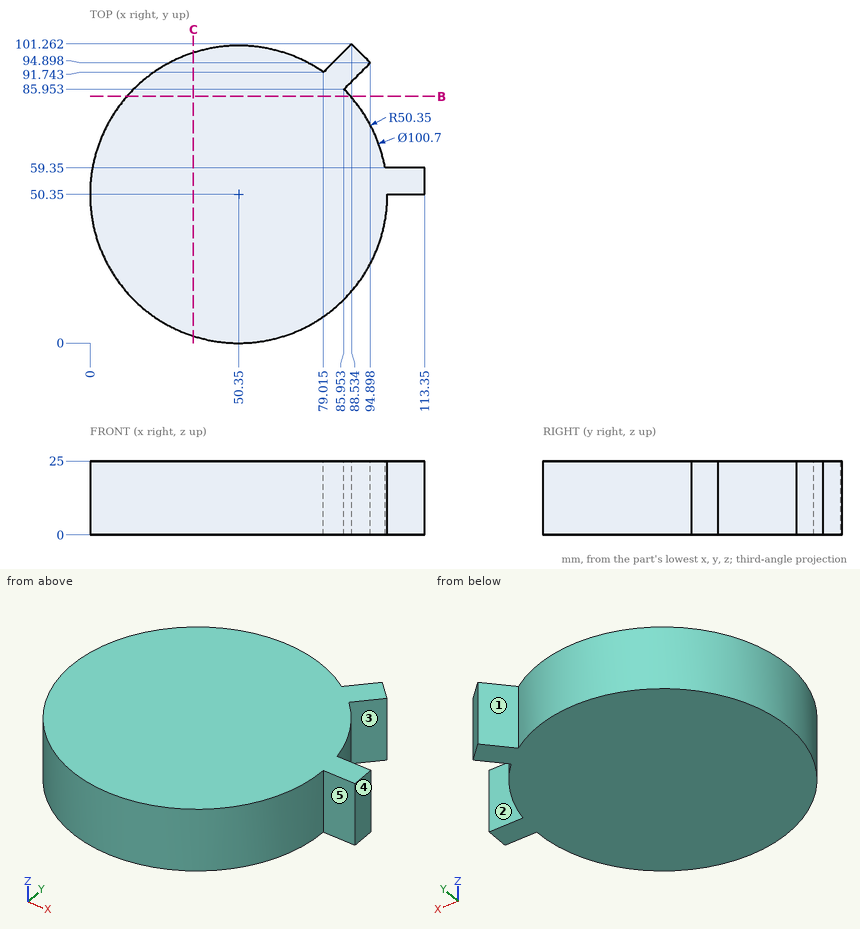
Verification items for this drawing (mm, ordinates from the low corner). A direction names the side the tool comes from. Give positions to 0.01 mm unless a question says otherwise; leave off trailing zeros. Loops run counter-clockwise (first coordinate to the right, second up) from the corner with the lowest first, then second, coordinate; pieces in that order, holes last. Notation, with made-up numbers: M -27,39 L 19,39 A19 cw 19,75 Z; hole C -38.75,87.25 d7. An arc over 180 degrees is marked long. Return JSON: item names as keys, results as strings. Group by question number.
1. Cross-section at C-C on x = 35. Record the boundary of the cut face in (y, z).
2. Mould release check, pull along X, two halves, no side actions. Record for the marked faces 1, 2 and 3: released by +X, released by -X, zero draft, split by the parting line, or undercut.
3. Go/stop test with flat-tipped pins: pin 1 (6.5 mm diameter, centred on x = 105, z = 7, fed in from -Y); pin 2 (12 mm diameter, centred on y = 39.5, z = 20, fed in from +X); pin 3 (1.5 mm diameter, centred on x = 60, z = 13.5, fed in from -Y). Record where each tip stops, or that it passes through.
4. Tool access check on the marked faces 4 and 5. Record the directions out of +Z, -Z, +X, -X, +Y, -Y that give a thin tool (end or side, any length) a straight path to the whole face; none if there is none.
5. Thickness scan on L1, parallel to Y at x = 105, z = 11; L2, parallel to Y at x = 14, z = 5.75; L3, parallel to X at y = 40, z = 12.5 (1 decimal). Record the ranges inside material, lowest first.
6. Cross-section at B-B on y = 83.5. Record the boundary of the cut face in (x, z).
Return value:
{
 "1": {"outline": "M 2.4,0 L 98.3,0 L 98.3,25 L 2.4,25 Z"},
 "2": {"face 1": "undercut", "face 2": "zero draft", "face 3": "released by +X"},
 "3": {"pin 1": "y = 50.35", "pin 2": "x = 100.47", "pin 3": "y = 0.79"},
 "4": {"face 4": "+Z, -Z, +X, +Y, -Y", "face 5": "+Z, -Z, +X, -Y"},
 "5": {"L1": "50.35 to 59.35", "L2": "15.51 to 85.19", "L3": "1.1 to 99.6"},
 "6": {"outline": "M 12.45,0 L 88.25,0 L 88.25,25 L 12.45,25 Z"}
}
